Verification items for the finished model (mm, model axes). Face numbers are marked on the shaded views. A direction names the side the tool comes from. Give positions to 0.01 mm unless a question says otherwise; leave off trailing zeros. Loops run counter-clockwise (first coordinate to the right, second up) from the corner with the lowest first, then second, coordinate; pieces in that order, holes last. Notation, with made-up numbers: (50, 77.5) - (57, 77.5) arc R10 ccw to (57, 90.5) - close; hole circle Ø10 at (81.25, 40). An arc over 180 degrees is marked (long way). Answer in a Markdown table with one row per item.
```python
from build123d import *

# Parameters (mm, degrees)
F4_W      = 206
F4_H      = 348
F5_DEPTH  = 1800
F6_T      = -2.5
F7_W      = 1062.3749792576
F7_H      = 600.0114679337
F8_DEPTH  = 391.7381567773
F9_W      = 166
F9_H      = 846
F10_DEPTH = 12.5


with BuildPart() as f5:
    # F4 (on face) → F5 (new body)
    with BuildSketch(Plane(origin=(1004.0916292849, 0, -1004.0916292849), x_dir=(0, 1, 0), z_dir=(0.7071067812, 0, -0.7071067812))):
        Rectangle(F4_W, F4_H)
    extrude(amount=-F5_DEPTH)

    # F6
    f6_openings = [f5.faces().sort_by_distance(p)[0] for p in [
        (1004.091629, 0, -1004.091629),
    ]]
    offset(amount=F6_T, openings=f6_openings)

    # F7 (on Top) → F8 (cut, through all)
    with BuildSketch(Plane.XY):
        with Locations((39.5732372999, -20.192950964)):
            Rectangle(F7_W, F7_H)
    extrude(amount=F8_DEPTH, mode=Mode.SUBTRACT)

    # F9 (on face) → F10 (cut, symmetric)
    with BuildSketch(Plane(origin=(123.0365799265, 0, 123.0365799265), x_dir=(0, 1, 0), z_dir=(0.7071067812, 0, 0.7071067812))):
        with Locations((0, -897)):
            Rectangle(F9_W, F9_H)
    extrude(amount=F10_DEPTH, both=True, mode=Mode.SUBTRACT)


solid = f5.part
```
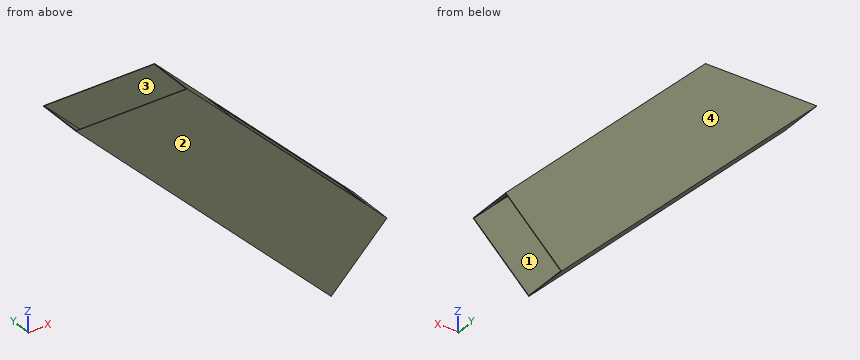
Q1. Thickness scan on line 1 (Y direction, x = 291.5, z = -86); line 2 (X direction, y = -6, z = -61.5); line 3 (Z direction, x = 257, y = -92). Record the ranges inside material, lowest first.
Completed:
| item | result |
|---|---|
| line 1 | -103 to -100.5, 100.5 to 103 |
| line 2 | -184.57 to -181.04, 304.04 to 307.57 |
| line 3 | -503.07 to -499.54, -14.46 to -10.93 |
Q2. Sectioned sample at C-C (x = 182). Record the cut outline in (y, z), and give its area (3 significant figures).
Completed:
| item | result |
|---|---|
| outline | (-103, -428.07) - (103, -428.07) - (103, 0) - (100.5, 0) - (100.5, -424.54) - (-100.5, -424.54) - (-100.5, 0) - (-103, 0) - close |
| area | 2,850 mm^2 |
Q3. Go/stop test with flat-tipped pins: P1, Ø5, axis at x = 689.5, y = 73, coming from the -Z side; P2, Ø6, axis at y = -2.5, z = -910.5, coming from the +X side; P3, Ø12, axis at y = 71, z = -140, coming from the +X side. Record where each tip stops, or that it passes through.
Completed:
| item | result |
|---|---|
| P1 | z = -938.07 |
| P2 | x = 670.96 |
| P3 | x = 392.07 |
Q4. Sectioned sample at B-B (z = -833). Record the cut outline in (x, y), and give its area (3 significant figures).
Completed:
| item | result |
|---|---|
| outline | (586.93, -103) - (1079.07, -103) - (1079.07, 103) - (586.93, 103) - close; hole (590.46, -100.5) - (1075.54, -100.5) - (1075.54, 100.5) - (590.46, 100.5) - close |
| area | 3,880 mm^2 |
Q5. Draft check along Z on the marked faces 3 and 4. Enter one of: +Z half, -Z half, draft (parallel to the pull), parting line (faces both ways), or undercut.
Completed:
| item | result |
|---|---|
| face 3 | undercut |
| face 4 | draft |
Q6. Sectioned sample at D-D (z = -245). Record the cut outline in (x, y), and give its area (3 significant figures).
Completed:
| item | result |
|---|---|
| outline | (-1.07, -103) - (491.07, -103) - (491.07, -83) - (487.54, -83) - (487.54, -100.5) - (2.46, -100.5) - (2.46, 100.5) - (487.54, 100.5) - (487.54, 83) - (491.07, 83) - (491.07, 103) - (-1.07, 103) - close |
| area | 3,300 mm^2 |
Q7. Tool access check on the marked faces 1 and 2. Record the directions out of +Z, -Z, +X, -X, +Y, -Y that give a thin tool (end or side, any length) a straight path to the whole face; none if there is none.
Completed:
| item | result |
|---|---|
| face 1 | none |
| face 2 | +Z, -Z, +X, -X, -Y |
Q8. Sectioned sample at A-A (y = -57.5). Record the cut outline in (x, z).
Completed:
| item | result |
|---|---|
| outline | (-246.07, 0) - (881.06, -1127.13) - (882.82, -1125.36) - (-242.54, 0) - close; (242.54, 0) - (456.44, -213.9) - (458.21, -212.13) - (246.07, 0) - close; (1054.65, -812.11) - (1125.36, -882.82) - (1127.13, -881.06) - (1056.42, -810.34) - close |
